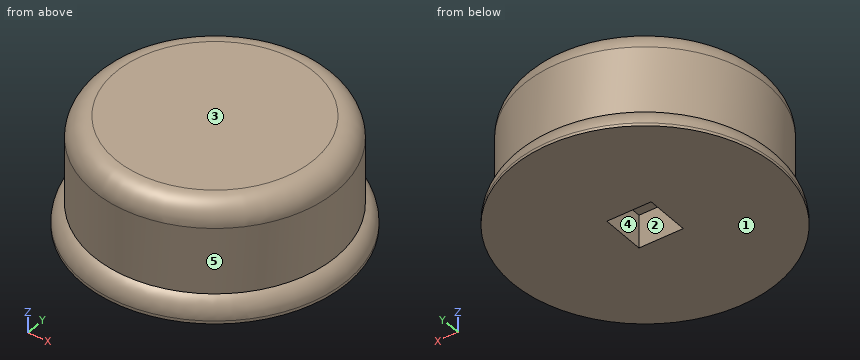
Autodesk Inventor part; units mm, degrees
ref_plane "YZ Plane" through (0, 0, 0) normal (1, 0, 0) x (0, 1, 0)
ref_plane "XZ Plane" through (0, 0, 0) normal (0, 1, 0) x (-1, 0, 0)
ref_plane "XY Plane" through (0, 0, 0) normal (0, 0, 1) x (1, 0, 0)
sketch "Sketch1" plane through (0, 0, 0) normal (0, 0, 1) x (1, 0, 0)
  circle A0 centre (0, 0) radius 6
  dimension "d0" = 12
extrude "Extrusion1" add sketch "Sketch1" along normal blind 1
sketch "Sketch2" plane through (0, 0, 1) normal (0, 0, 1) x (1, 0, 0)
  circle A0 centre (0, 0) radius 5.5
  dimension "d3" = 11
extrude "Extrusion2" add sketch "Sketch2" along normal blind 4
fillet "Fillet1" radius 1 1 edges at (-6, 0, 1)
fillet "Fillet2" radius 1 1 edges at (-5.5, 0, 5)
sketch "Sketch3" plane through (0, 0, 0) normal (0, 0, -1) x (-1, 0, 0)
  line L0 (0, -1) -> (1, -1)
  line L1 (1, -1) -> (1, 1)
  line L2 (1, 1) -> (-1, 1)
  line L3 (-1, 1) -> (-1, -1)
  line L4 (-1, -1) -> (0, -1)
  point P0 (0, 0)
  dimension "d8" = 1
  dimension "d9" = 2
  dimension "d10" = 1
  dimension "d13" = 1
extrude "Extrusion3" cut sketch "Sketch3" against normal blind 1.5
sketch "Sketch4" plane through (0, 0, 0) normal (0, 0, -1) x (-1, 0, 0)
  point P0 (0, 0)
properties part number "BTN_3"
Geometry: final body of the model. Coordinates: model frame, mm. Face numbers are marked on the shaded views. A direction names the side the tool comes from. Coordinates: 2 decimals unless noted, no trailing zeros. Order: outer loops, then holes, each group sorted by start corner. A loop starts at its lowest first (then second) coordinate and runs counter-clockwise, first axis right, second up.
1) Section D-D (z = 2.8). Return loops of the section in (x, y), then the cut area to 3 significant figures.
Result sheet:
outline: circle Ø11 at (0, 0)
area: 95.0 mm2
2) Section A-A (z = 1.3). Return loops of the section in (x, y), then the cut area to 3 significant figures.
Result sheet:
outline: circle Ø11 at (0, 0); hole (-1, -1) - (1, -1) - (1, 1) - (-1, 1) - close
area: 91.0 mm2
3) Ray query, probe 1 along Z at (x, y) = (-4, -2.25); probe 2 along X at (y, z) = (-0.75, 4.25); probe 3 along X at (y, z) = (-1.5, 0.5). Return the intervals inside material, ascending.
Result sheet:
probe 1: z = 0 to 5
probe 2: x = -5.42 to 5.42
probe 3: x = -5.74 to 5.74
4) Set-up query: the marked faces 1 and 2. Return all of +Z, -Z, +X, -X, +Y, -Y with unobstructed straight access to the full face (end or side cutting, diameter ignored); none if empty.
Result sheet:
face 1: -Z, +X, -X, +Y, -Y
face 2: -Z
5) Draft query along X for the marked faces 3, 4 and 5. Return one class per face: released by +X, released by -X, zero draft, split by the parting line, or undercut.
Result sheet:
face 3: zero draft
face 4: undercut
face 5: split by the parting line
6) First-contact query: P1, Ø1, axis at y = -3.5, z = 1.5, coming from the +X side; P2, Ø2, axis at x = 4.5, z = 2.5, coming from the +Y side; P3, Ø1.5, axis at y = 4, z = 1, coming from the -X side. Flat tips, straight axial feed; report the tip coordinate or a pass-through.
Result sheet:
P1: stops at x = 4.61
P2: stops at y = 4.24
P3: stops at x = -4.83
7) Section B-B (y = 0). Return loops of the section in (x, z), then the cut area to 3 significant figures.
Result sheet:
outline: (-6, 0) - (-1, 0) - (-1, 1.5) - (1, 1.5) - (1, 0) - (6, 0) - (6, 0.13) arc R1 ccw to (5.5, 1) - (5.5, 4) arc R1 ccw to (4.5, 5) - (-4.5, 5) arc R1 ccw to (-5.5, 4) - (-5.5, 1) arc R1 ccw to (-6, 0.13) - close
area: 52.3 mm2
